```python
from build123d import *

# Parameters (mm, degrees)
F1_DEPTH = 10
F2_R     = 3
F4_DEPTH = 8
F5_R     = 0.65
F6_DEPTH = 7


with BuildPart() as f1:
    # F0 (on Top) → F1 (new body)
    with BuildSketch(Plane.XY):
        with BuildLine():
            ThreePointArc((0, 8), (2.343146, 2.343146), (8, 0))
            Line((8, 0), (27, 0))
            Line((27, 0), (27, 21))
            ThreePointArc((27, 21), (22.757359, 22.757359), (21, 27))
            Line((21, 27), (0, 27))
            Line((0, 27), (0, 8))
        make_face()
    extrude(amount=F1_DEPTH)

    # F2
    f2_edges = [f1.edges().sort_by_distance(p)[0] for p in [
        (17.5, 0, 0),
        (2.343146, 2.343146, 0),
        (0, 17.5, 0),
    ]]
    fillet(f2_edges, radius=F2_R)

    # F3 (on face) → F4 (cut)
    with BuildSketch(Plane.XY.offset(10)):
        with BuildLine():
            Line((20.071797, 26), (1, 26))
            Line((1, 26), (1, 8))
            ThreePointArc((1, 8), (3.050253, 3.050253), (8, 1))
            Line((8, 1), (26, 1))
            Line((26, 1), (26, 20.071797))
            ThreePointArc((26, 20.071797), (22.050253, 22.050253), (20.071797, 26))
        make_face()
        with BuildLine():
            Line((1, 27), (1, 26))
            Line((1, 26), (20.071797, 26))
            ThreePointArc((20.071797, 26), (22.050253, 22.050253), (26, 20.071797))
            Line((26, 20.071797), (26, 1))
            Line((26, 1), (27, 1))
            Line((27, 1), (27, 21))
            ThreePointArc((27, 21), (22.757359, 22.757359), (21, 27))
            Line((21, 27), (1, 27))
        make_face()
    extrude(amount=-F4_DEPTH, mode=Mode.SUBTRACT)

    # F5 (on face) → F6 (join)
    with BuildSketch(Plane.XY.offset(2)):
        with Locations((21, 5)):
            Circle(F5_R)
        with BuildLine():
            ThreePointArc((5.65, 21), (5.459619, 21.459619), (5, 21.65))
            ThreePointArc((5, 21.65), (4.540381, 20.540381), (5.65, 21))
        make_face()
    extrude(amount=F6_DEPTH)


solid = f1.part
```
Part model, mm, in its own coordinate system. A direction names the side the tool comes from. Round coordinates to 2 decimals unless told otherwise and drop trailing zeros. Loops run counter-clockwise (first coordinate to the right, second up) from the corner with the lowest first, then second, coordinate; pieces in that order, holes last.
Item 1: Drop flat-ended pins along their axis: P1, Ø2, axis at x = 4, y = 15, coming from the +Z side; P2, Ø1.4, axis at x = 21.5, y = 5, coming from the +Z side; P3, Ø4, axis at y = 13.5, z = 5, coming from the +X side. Give the stop position or say it passes through.
Item 2: Cut at D-D, the plane z = 1. Give the cut face in (x, y).
Item 3: 3-axis set-ups, long thin cutter, end or side, ignore diameter. For faces 5 (the face through (1, 6, 10)), 6 (the face through (21, 5, 9)): which of +Z, -Z, +X, -X, +Y, -Y reach the whole face in a straight line?
Item 4: Cut at B-B, the plane x = 9.5. Give the cut face in (y, z), then the cut area to 3 significant figures.
Item 5: Cut at A-A, the plane z = 5. Give the cut face in (x, y), then the cut area to 3 significant figures.
Item 6: Mould opens along Y. For faces 1 (the face through (15, 15, 0)), 2 (the face through (2.281, 2.406, 6.451)), 3 (the face through (22.804, 22.711, 0.986)), 4 (the face through (20.35, 5.03, 5.45)) say: +Y half, -Y half, draft (parallel to the pull), parting line (faces both ways), or undercut.
Item 7: Drill centre lines: line 1 (Y direction, x = 21, z = 4.75); line 2 (Y direction, x = 25.5, z = 4). Where is each one in solid material? Low to high.
A:
1. P1: stops at z = 2
1. P2: stops at z = 9
1. P3: stops at x = 1
2. outline: (0.76, 8) arc R7.24 ccw to (8, 0.76) - (27, 0.76) - (27, 21) arc R6 cw to (21, 27) - (0.76, 27) - close
3. face 5: +Z, +X, -X, +Y, -Y
3. face 6: +Z, +X, +Y
4. outline: (0, 3) arc R3 ccw to (3, 0) - (27, 0) - (27, 2) - (1, 2) - (1, 10) - (0, 10) - close
4. area: 60.1 mm2
5. outline: (0, 8) arc R8 ccw to (8, 0) - (27, 0) - (27, 1) - (8, 1) arc R7 cw to (1, 8) - (1, 27) - (0, 27) - close; (5, 21.65) arc R0.65 ccw (long way) to (5.65, 21) arc R0.65 ccw to start; circle Ø1.3 at (21, 5)
5. area: 52.4 mm2
6. face 1: draft
6. face 2: -Y half
6. face 3: +Y half
6. face 4: undercut
7. line 1: y = 0 to 1, 4.35 to 5.65
7. line 2: y = 0 to 1
